Input: part model. Units: mm. Frame: model coordinates. Round coordinates to 2 decimals unless told otherwise and drop trailing zeros. Loops run counter-clockwise (first coordinate to the right, second up) from the corner with the lowest first, then second, coordinate; pieces in that order, holes last. Notation, with made-up numbers: (-16, 60) - (27, 60) arc R19 ccw to (27, 76) - close; hole circle Ø4 at (-30, 1.5). An arc over 180 degrees is marked (long way). Use CSV: the item, a comma, the result in double quotes. Start each with the question number.
1. Cut plane C-C (z = 0.2). Give the number of separate pieces and of enclosed holes in the cut face, and give its area (3 significant figures).
2. Pin query (flat end, axial travel): P1, Ø12, axis at x = 70, y = 63.5, coming from the -Z side. Return the tip coordinate at first contact, or that it passes through.
3. Cut plane A-A (y = 34). Return loops of the section in (x, z).
4. Material intervals for probe 1 along X at (y, z) = (51.5, 0.2); probe 2 along X at (y, z) = (12.5, 0.2); probe 3 along Y at (x, z) = (42.5, 0.15), sorted ascending. Write a range as from..to.
5. Cut plane B-B (x = 91). Return loops of the section in (y, z), and give its area (3 significant figures).
```python
from build123d import *

# Parameters (mm, degrees)
BOSS_EXTRUDE1_DEPTH = 0.254
SKETCH2_R           = 4.699
CUT_EXTRUDE1_DEPTH  = 1.254
SKETCH3_W           = 2.54
SKETCH3_H           = 0.635
CUT_EXTRUDE2_DEPTH  = 1.254
CUT_EXTRUDE4_DEPTH  = 1.254
CUT_EXTRUDE5_DEPTH  = 1.254


with BuildPart() as part:
    # Sketch1 → Boss-Extrude1 (new body)
    with BuildSketch(Plane.XY):
        with BuildLine():
            Line((67.21146711, 76.191723231), (8.696654013, 17.676910134))
            Line((8.696654013, 17.676910134), (7.228954972, 14.133571205))
            ThreePointArc((7.228954972, 14.133571205), (14.666587579, 6.075099489), (15.105587123, -4.88230096))
            Line((15.105587123, -4.88230096), (18.648926052, -6.35))
            Line((18.648926052, -6.35), (101.401368334, -6.35))
            ThreePointArc((101.401368334, -6.35), (93.866160503, 38.880636728), (67.21146711, 76.191723231))
        make_face()
        with BuildLine():
            Line((88.672924278, 6.35), (27.86051193, 6.35))
            ThreePointArc((27.86051193, 6.35), (26.399857642, 10.93517908), (24.190484974, 15.210228852))
            Line((24.190484974, 15.210228852), (67.191354125, 58.211098004))
            ThreePointArc((67.191354125, 58.211098004), (82.13289044, 34.020557137), (88.672924278, 6.35))
        make_face(mode=Mode.SUBTRACT)
    extrude(amount=BOSS_EXTRUDE1_DEPTH)

    # Sketch2 → Cut-Extrude1 (cut, through all)
    with BuildSketch(Plane.XY.offset(0.254)):
        with Locations((22.225, 0)):
            Circle(SKETCH2_R)
        with Locations((36.195, 0)):
            Circle(SKETCH2_R)
        with Locations((61.722, 0)):
            Circle(SKETCH2_R)
        with Locations((75.692, 0)):
            Circle(SKETCH2_R)
        with Locations((95.25, 0)):
            Circle(SKETCH2_R)
        with Locations((15.715448212, 15.715448212)):
            Circle(SKETCH2_R)
        with Locations((25.593729945, 25.593729945)):
            Circle(SKETCH2_R)
        with Locations((43.644044748, 43.644044748)):
            Circle(SKETCH2_R)
        with Locations((53.522326482, 53.522326482)):
            Circle(SKETCH2_R)
        with Locations((92.004434954, 24.652514046)):
            Circle(SKETCH2_R)
        with Locations((82.48891971, 47.625)):
            Circle(SKETCH2_R)
        with Locations((67.351920908, 67.351920908)):
            Circle(SKETCH2_R)
    extrude(amount=-CUT_EXTRUDE1_DEPTH, mode=Mode.SUBTRACT)

    # Sketch3 → Cut-Extrude2 (cut, through all)
    with BuildSketch(Plane.XY.offset(0.254)):
        Polygon((15.266435406, 24.246691527), (17.06248663, 26.042742751), (17.511499436, 25.593729945), (15.715448212, 23.797678721), align=None)
        Polygon((44.991083167, 53.971339288), (43.195031942, 52.175288063), (43.644044748, 51.726275257), (45.440095973, 53.522326482), align=None)
        with Locations((29.21, -6.0325)):
            Rectangle(SKETCH3_W, SKETCH3_H)
        with Locations((68.707, -6.0325)):
            Rectangle(SKETCH3_W, SKETCH3_H)
        Polygon((29.230733674, 38.210989795), (31.026784898, 40.007041019), (31.475797704, 39.558028213), (29.67974648, 37.761976989), align=None)
        Polygon((56.845021246, 65.825277367), (55.048970022, 64.029226143), (55.497982828, 63.580213337), (57.294034052, 65.376264561), align=None)
        with Locations((48.9585, -6.0325)):
            Rectangle(SKETCH3_W, SKETCH3_H)
        with Locations((85.471, -6.0325)):
            Rectangle(SKETCH3_W, SKETCH3_H)
        Polygon((99.935462164, 14.437711971), (100.266998693, 11.919442024), (101.526133667, 12.085210288), (101.194597138, 14.603480236), align=None)
        Polygon((93.765504959, 37.464305742), (94.938831965, 37.950313702), (93.966816047, 40.296967714), (92.793489041, 39.810959755), align=None)
        Polygon((79.327792988, 62.471156422), (80.874047017, 60.456038938), (81.88160576, 61.229165953), (80.33535173, 63.244283437), align=None)
        Polygon((13.593916116, 7.005422516), (14.565932035, 4.658768503), (15.739259041, 5.144776462), (14.767243123, 7.491430475), align=None)
    extrude(amount=-CUT_EXTRUDE2_DEPTH, mode=Mode.SUBTRACT)

    # Sketch6 → Cut-Extrude4 (cut, through all)
    with BuildSketch(Plane.XY.offset(0.254)):
        with BuildLine():
            Line((22.27103518, 28.91642471), (40.321349984, 46.966739513))
            ThreePointArc((40.321349984, 46.966739513), (46.966739513, 46.966739513), (46.966739513, 40.321349984))
            Line((46.966739513, 40.321349984), (28.91642471, 22.27103518))
            ThreePointArc((28.91642471, 22.27103518), (22.27103518, 22.27103518), (22.27103518, 28.91642471))
        make_face()
        with BuildLine():
            Line((50.199631717, 56.845021246), (64.029226143, 70.674615673))
            ThreePointArc((64.029226143, 70.674615673), (70.674615673, 70.674615673), (70.674615673, 64.029226143))
            Line((70.674615673, 64.029226143), (56.845021246, 50.199631717))
            ThreePointArc((56.845021246, 50.199631717), (50.199631717, 50.199631717), (50.199631717, 56.845021246))
        make_face()
        with BuildLine():
            Line((61.722, -4.699), (36.195, -4.699))
            ThreePointArc((36.195, -4.699), (31.496, 0), (36.195, 4.699))
            Line((36.195, 4.699), (61.722, 4.699))
            ThreePointArc((61.722, 4.699), (66.421, 0), (61.722, -4.699))
        make_face()
        with BuildLine():
            Line((95.25, -4.699), (75.692, -4.699))
            ThreePointArc((75.692, -4.699), (70.993, 0), (75.692, 4.699))
            Line((75.692, 4.699), (95.25, 4.699))
            ThreePointArc((95.25, 4.699), (99.949, 0), (95.25, -4.699))
        make_face()
        with BuildLine():
            ThreePointArc((26.924, 0), (24.874532533, 10.303368733), (19.038142977, 19.038142977))
            ThreePointArc((19.038142977, 19.038142977), (12.392753447, 19.038142977), (12.392753447, 12.392753447))
            ThreePointArc((12.392753447, 12.392753447), (16.191912687, 6.706909836), (17.526, 0))
            ThreePointArc((17.526, 0), (22.225, -4.699), (26.924, 0))
        make_face()
    extrude(amount=-CUT_EXTRUDE4_DEPTH, mode=Mode.SUBTRACT)

    # Sketch5 → Cut-Extrude5 (cut, through all)
    with BuildSketch(Plane.XY.offset(0.254)):
        with BuildLine():
            Line((81.390083385, 32.475702096), (95.471027857, 38.308220267))
            ThreePointArc((95.471027857, 38.308220267), (99.36478975, 26.62471517), (101.834445583, 14.559622003))
            Line((101.834445583, 14.559622003), (86.723730875, 12.570258672))
            ThreePointArc((86.723730875, 12.570258672), (84.644080158, 22.680312922), (81.390083385, 32.475702096))
        make_face()
    extrude(amount=-CUT_EXTRUDE5_DEPTH, mode=Mode.SUBTRACT)


solid = part.part
```
Established:
1,separate pieces,"1"
1,enclosed holes,"6"
1,area,"1,290 mm2"
2,P1,"stops at z = 0"
3,outline,"(25.02, 0) - (27.35, 0) - (27.35, 0.25) - (25.02, 0.25) - close; (40.65, 0) - (42.98, 0) - (42.98, 0.25) - (40.65, 0.25) - close; (82.14, 0) - (85.07, 0) - (85.07, 0.25) - (82.14, 0.25) - close"
4,probe 1,"x = 42.52..49.28, 58.15..60.48, 72.46..79.83, 85.15..87.58"
4,probe 2,"x = 9.79..12.29, 23.85..25.7, 88.02..100.19"
4,probe 3,"y = -6.35..-4.7, 4.7..6.35, 33.52..35.85, 48.2..51.48"
5,outline,"(-6.35, 0) - (-4.7, 0) - (-4.7, 0.25) - (-6.35, 0.25) - close; (4.7, 0) - (13.13, 0) - (13.13, 0.25) - (4.7, 0.25) - close; (36.46, 0) - (45.18, 0) - (45.18, 0.25) - (36.46, 0.25) - close"
5,area,"4.78 mm2"
